The drawing under review shows one solid part. Ordinate dimensions are in mm from its lowest x, y, z. A direction names the side the tool comes from. Round coordinates to 2 decimals unless told otherwise and drop trailing zeros. Write each loop counter-clockwise with the first axis right and the second up, starting at its lowest first coordinate (ties: lowest second). Pieces come first, ordered by that corner, then holes. Notation, with made-up numbers: M 16,10.5 L 65,10.5 A14 cw 65,28.5 Z; hole C 3,48.5 d7. An arc over 180 degrees is marked long. One line per item, written item: value. Start each with the question number.
1) Take a section at D-D, the plane x = 3.5. Write out the cut boundary in (y, z).
2) Mouldability with a two-part tool opening along X and no side actions: class the marked faces 1, 2, 3 and 4 as +X half, -X half, draft (parallel to the pull), parting line (faces both ways), or undercut.
3) Take a section at B-B, the plane z = 10.25. Write out the cut boundary in (x, y), and give its area (3 significant figures).
4) Wall thickness on probe 1 along X at (y, z) = (9.75, 8.5) (1 decimal); probe 2 along X at (y, z) = (17, 14.5); probe 3 along X at (y, z) = (4.5, 16): over which ranges is each line inside the solid? List them lowest first.
5) Take a section at C-C, the plane y = 4. Write out the cut boundary in (x, z), and give its area (3 significant figures).
6) Take a section at A-A, the plane y = 16.5. Write out the cut boundary in (x, z).
7) Tool access review of the marked faces 5, 6 and 7: name each direction out of +Z, -Z, +X, -X, +Y, -Y from which nothing blocks a thin tool from reaching the whole face with its end or side.
8) For P1, Ø2, axis at x = 3.5, y = 12.5, coming from the +Z side; P2, Ø2.5, axis at y = 2, z = 18.5, coming from the +X side, all flat-tipped, find the tip position at first contact; note any pin that passes through.
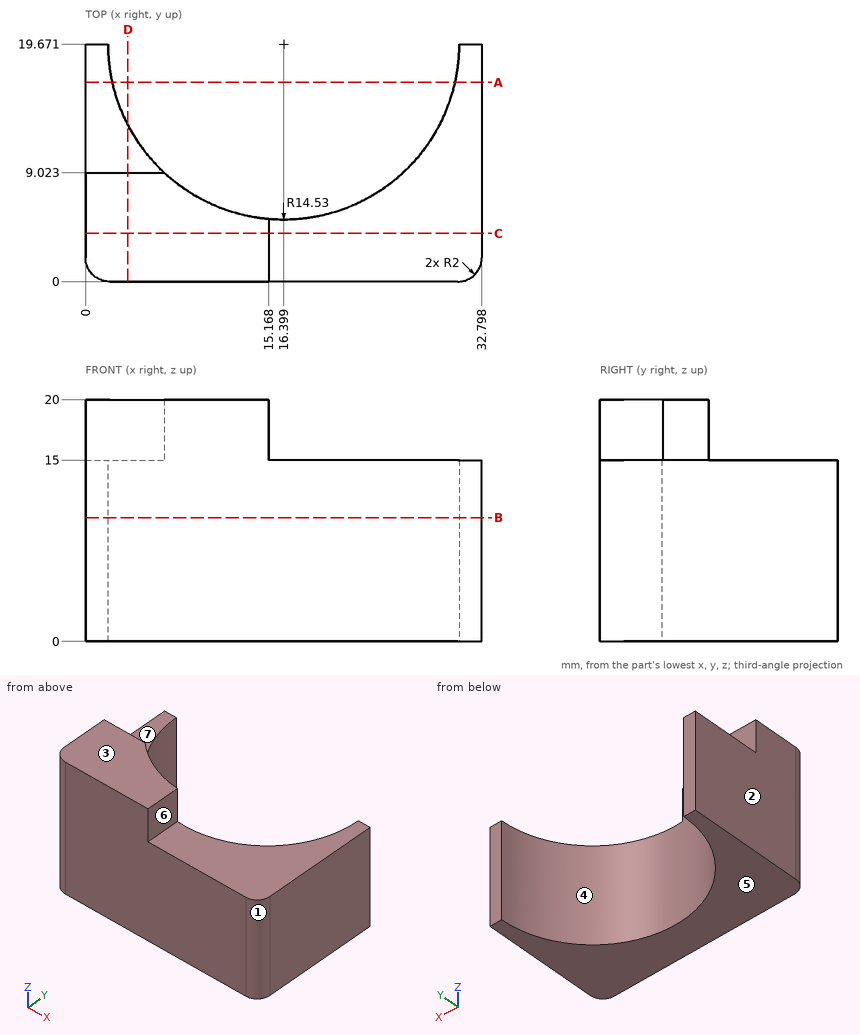
Checked values:
1. outline: M 0,0 L 12.98,0 L 12.98,15 L 9.02,15 L 9.02,20 L 0,20 Z
2. face 1: +X half
2. face 2: -X half
2. face 3: draft
2. face 4: undercut
3. outline: M 0,2 A2 ccw 2,0 L 30.8,0 A2 ccw 32.8,2 L 32.8,19.67 L 30.93,19.67 A14.53 cw 1.87,19.67 L 0,19.67 Z
3. area: 312 mm2
4. probe 1: x = 0 to 5.8, 27 to 32.8
4. probe 2: x = 0 to 2.12, 30.68 to 32.8
4. probe 3: x = 0 to 15.17
5. outline: M 0,0 L 32.8,0 L 32.8,15 L 15.17,15 L 15.17,20 L 0,20 Z
5. area: 568 mm2
6. outline: M 0,0 L 2.22,0 L 2.22,15 L 0,15 Z; M 30.58,0 L 32.8,0 L 32.8,15 L 30.58,15 Z
7. face 5: -Z, +X, -X, +Y, -Y
7. face 6: +Z, +X, +Y, -Y
7. face 7: +Z, +X, -X, +Y
8. P1: stops at z = 15
8. P2: stops at x = 15.17
